For this review, take the finished solid that the model builds, in its own axes (mm). A direction names the side the tool comes from. Coordinates: 2 decimals unless noted, no trailing zeros. Loops run counter-clockwise (first coordinate to the right, second up) from the corner with the lowest first, then second, coordinate; pieces in that order, holes last. Notation, with made-up numbers: (23, -34.75) -> (35, -34.75) arc R19 cw to (35, -10.75) -> close; hole circle Ø11 at (-1.5, 70.5). An arc over 180 degrees is marked (long way). Use a Markdown table: item, result.
from build123d import *

# Parameters (mm, degrees)
F0_W     = 152.4
F0_H     = 152.4
F1_DEPTH = 2.032
F2_W     = 148.336
F2_H     = 148.336
F3_DEPTH = 8.636
F4_W     = 148.336
F4_H     = 148.336
F5_DEPTH = 2.032


with BuildPart() as f1:
    # F0 (on Right) → F1 (new body)
    with BuildSketch(Plane.YZ):
        with Locations((76.2, 76.2)):
            Rectangle(F0_W, F0_H)
    extrude(amount=F1_DEPTH)

    # F2 (on face) → F3 (join)
    with BuildSketch(Plane.YZ.offset(2.032)):
        with Locations((76.2, 76.2)):
            Rectangle(F2_W, F2_H)
    extrude(amount=F3_DEPTH)

    # F4 (on face) → F5 (join)
    with BuildSketch(Plane.YZ.offset(10.668)):
        Polygon((0, 152.4), (0, 2.032), (0, 0), (152.4, 0), (152.4, 152.4), align=None)
        with Locations((76.2, 76.2)):
            Rectangle(F4_W, F4_H, mode=Mode.SUBTRACT)
        with Locations((76.2, 76.2)):
            Rectangle(F4_W, F4_H)
    extrude(amount=F5_DEPTH)


solid = f1.part
(1) For line 1 along Y through (x, z) = (10.5, 138.5), list the stretches that pass through material, from the lowest coordinate up.
Found:
| item | result |
|---|---|
| line 1 | y = 2.03 to 150.37 |
(2) Take a section at A-A on y = 48.5. Write out the cut boundary in (x, z), plus the area to 3 significant figures.
Found:
| item | result |
|---|---|
| outline | (0, 0) -> (2.03, 0) -> (2.03, 2.03) -> (10.67, 2.03) -> (10.67, 0) -> (12.7, 0) -> (12.7, 152.4) -> (10.67, 152.4) -> (10.67, 150.37) -> (2.03, 150.37) -> (2.03, 152.4) -> (0, 152.4) -> close |
| area | 1,900 mm^2 |
(3) Mouldability with a two-part tool opening along X and no side actions: class faces 4 (the face through (12.7, 75, 77)), 5 (the face through (6, 2.032, 75)), 6 (the face through (0, 75, 77)) as pulls with the +X half, pulls with the -X half, needs draft (parallel to the pull), parting line crosses it, or undercut.
Found:
| item | result |
|---|---|
| face 4 | pulls with the +X half |
| face 5 | undercut |
| face 6 | pulls with the -X half |
(4) Take a section at C-C on x = 7.5. Write out the cut boundary in (y, z).
Found:
| item | result |
|---|---|
| outline | (2.03, 2.03) -> (150.37, 2.03) -> (150.37, 150.37) -> (2.03, 150.37) -> close |
(5) For pin 1 Ø3 at (x, z) = (5.5, 107) entering from -Y; pin 2 Ø7 at (x, y) = (6.5, 41.5) entering from +Z; pin 3 Ø2.5 at (x, y) = (6.5, 97) entering from -Z, all flat-tipped, find the tip position at first contact; note any pin that passes through.
Found:
| item | result |
|---|---|
| pin 1 | stops at y = 2.03 |
| pin 2 | stops at z = 150.37 |
| pin 3 | stops at z = 2.03 |
(6) For faces 1 (the face through (6, 75, 150.368)), 2 (the face through (6, 150.368, 75)), 3 (the face through (6, 75, 2.032)), list the 3-axis set-ups (+Z, -Z, +X, -X, +Y, -Y) from which the entire face can be reached by the end or side of a thin tool; tool diameter is ignored.
Found:
| item | result |
|---|---|
| face 1 | +Z, +Y, -Y |
| face 2 | +Z, -Z, +Y |
| face 3 | -Z, +Y, -Y |
